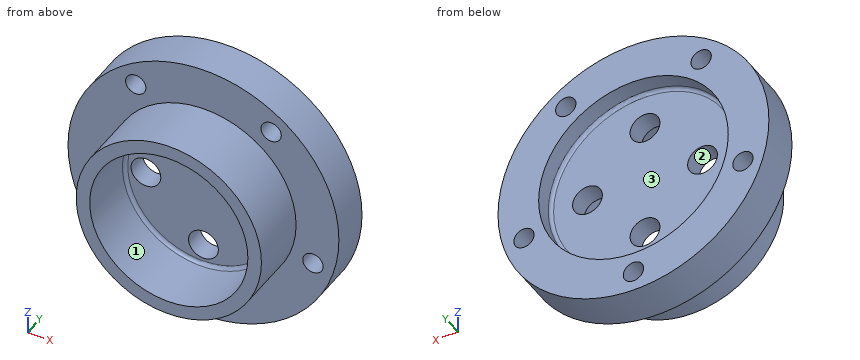
```python
from build123d import *

# Parameters (mm, degrees)
SKETCH2_R          = 3.4925
CUT_EXTRUDE1_DEPTH = 20.05
SKETCH3_R          = 2.38125
CUT_EXTRUDE2_DEPTH = 24.8125
CIRPATTERN1_COUNT  = 5
FILLET1_R          = 0.79375


with BuildPart() as part:
    # Sketch1 → Revolve1 (revolve)
    with BuildSketch(Plane.XY):
        Polygon((18.542, -14.2875), (18.542, 0), (0, 0), (0, 4.7625), (22.225, 4.7625), (22.225, 9.525), (31.75, 9.525), (31.75, 0), (21.717, 0), (21.717, -14.2875), align=None)
    revolve(axis=Axis((0, 0, 0), (0, 1, 0)))

    # Sketch2 → Cut-Extrude1 (cut, through all)
    with BuildSketch(Plane(origin=(0, 4.7625, 0), x_dir=(1, 0, 0), z_dir=(0, 1, 0))):
        with Locations((-13.4874, 0)):
            Circle(SKETCH2_R)
        with Locations((0, 13.4874)):
            Circle(SKETCH2_R)
        with Locations((13.4874, 0)):
            Circle(SKETCH2_R)
        with Locations((0, -13.4874)):
            Circle(SKETCH2_R)
    extrude(amount=-CUT_EXTRUDE1_DEPTH, mode=Mode.SUBTRACT)

    # Sketch3 → Cut-Extrude2 (cut, through all)
    with BuildSketch(Plane(origin=(0, 9.525, 0), x_dir=(1, 0, 0), z_dir=(0, 1, 0))):
        with Locations((0, 26.9875)):
            Circle(SKETCH3_R)
    cut_extrude2 = extrude(amount=-CUT_EXTRUDE2_DEPTH, mode=Mode.SUBTRACT)

    # CirPattern1: Cut-Extrude2 ×5 about axis
    cirpattern1_axis = Axis((0, 0, 0), (0, 1, 0))
    for i in range(1, CIRPATTERN1_COUNT):
        add(cut_extrude2.rotate(cirpattern1_axis, i * 360 / CIRPATTERN1_COUNT), mode=Mode.SUBTRACT)

    # Fillet1
    fillet1_edges = [part.edges().sort_by_distance(p)[0] for p in [
        (-18.542, 0, 0),
        (-22.225, 4.7625, 0),
    ]]
    fillet(fillet1_edges, radius=FILLET1_R)


solid = part.part
```
Source: CAD feature listing. Evaluate the final solid. Frame: model axes, mm. Face numbers are marked on the shaded views. A direction names the side the tool comes from. Round coordinates to 2 decimals unless told otherwise and drop trailing zeros. Order: outer loops, then holes, each group sorted by start corner. A loop starts at its lowest first (then second) coordinate and runs counter-clockwise, first axis right, second up. Notation, with made-up numbers: (-24, 59.25) -> (20, 59.25) arc R25 ccw to (20, 94.25) -> close; hole circle Ø5 at (78.5, -11.75). An arc over 180 degrees is marked (long way). Use CSV: the item, a comma, the result in double quotes.
(1) Ray query, L1, parallel to Z at x = 0, y = 3; L2, parallel to X at y = 6.4, z = 0 (3 decimals); L3, parallel to Z at x = -0.5, y = -5. Return the intervals inside material, ascending.
Report:
L1,"-31.75 to -29.37, -24.61 to -16.98, -9.99 to 9.99, 16.98 to 31.75"
L2,"-31.75 to -22.225, 22.225 to 31.75"
L3,"-21.71 to -18.54, 18.54 to 21.71"
(2) First-contact query: pin 1 Ø7.5 at (x, z) = (-15.86, 21.83) entering from -Y; pin 2 Ø12 at (y, z) = (-7.5, -13) entering from -X; pin 3 Ø12 at (y, z) = (-1.5, -8) entering from -X; pin 4 Ø5.5 at (x, z) = (13.49, 0) entering from -Y. Flat tips, straight axial feed; report the tip coordinate or a pass-through.
Report:
pin 1,"y = 0"
pin 2,"x = -20.56"
pin 3,"x = -31.67"
pin 4,"through"
(3) Section A-A on x = 0. Count the separate pieces of the cut face and the enclosed holes in it, and give its area (3 significant figures).
Report:
separate pieces,"4"
enclosed holes,"0"
area,"373 mm^2"
(4) Section D-D on y = -5. Return the cut outline in (x, z), and give its area (3 significant figures).
Report:
outline,"circle Ø43.43 at (0, 0); hole circle Ø37.08 at (0, 0)"
area,"402 mm^2"
(5) Access query for the marked faces 1, 2 and 3. Directions: +Z, -Z, +X, -X, +Y, -Y. A direction counts if a zero-diameter tool reaches every point of the face in a straight line with its end or side. Return the directions, or none.
Report:
face 1,"-Y"
face 2,"+Y, -Y"
face 3,"+Y"
